Geometry check sheet. Reference: the model listing, model coordinates, mm. Face numbers are marked on the shaded views. A direction names the side the tool comes from. Round coordinates to 2 decimals unless told otherwise and drop trailing zeros. Loops run counter-clockwise (first coordinate to the right, second up) from the corner with the lowest first, then second, coordinate; pieces in that order, holes last. Notation, with made-up numbers: M 2,26.5 L 39,26.5 A30 ccw 39,59.5 Z; hole C -32.5,-36.5 d9. An arc over 180 degrees is marked long. Use one line per item in the form item = value. Start each with the question number.
1. Material ranges on line 1 (Y direction, x = -5, z = 0); line 2 (Y direction, x = -14, z = -3); line 3 (Y direction, x = -15.5, z = 13), recorded low to high.
2. Go/stop test with flat-tipped pins: pin 1 (4 mm diameter, centred on x = -11, y = 40.5, fed in from +Z); pin 2 (6 mm diameter, centred on y = 45, z = -4, fed in from -X); pin 3 (6.5 mm diameter, centred on x = -2.5, y = 44, fed in from -Z). Record where each tip stops, or that it passes through.
3. Cross-section at B-B (x = 15). Record the boundary of the cut face in (y, z).
4. Draft check along Y on the marked faces 1, 2, 3 and 4. Enter one of: pulls with the +Y half, pulls with the -Y half, needs draft (parallel to the pull), parting line crosses it, or undercut.
5. Cross-section at A-A (z = 0.5). Record the boundary of the cut face in (x, y), then the cut area to 3 significant figures.
6. Cross-section at D-D (z = -11.5). Record the boundary of the cut face in (x, y), then the cut area to 3 significant figures.
7. Set-up check for the marked faces 5, 6 and 7: record each of +Z, -Z, +X, -X, +Y, -Y from which the full face is reachable in a straight line by a thin tool's end or side.
8. Cross-section at C-C (y = 13.5). Record the boundary of the cut face in (x, z), then the cut area to 3 significant figures.
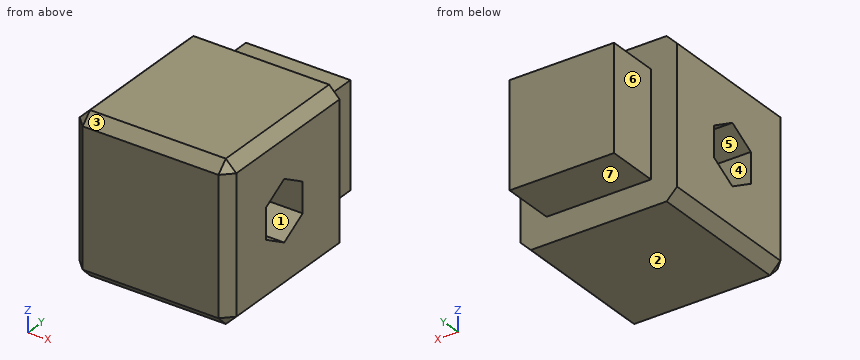
```python
from build123d import *

# Parameters (mm, degrees)
SKETCH1_W           = 38.1
SKETCH1_H           = 38.1
BOSS_EXTRUDE1_DEPTH = 50.8
SKETCH2_W           = 38.1
SKETCH2_H           = 38.1
SKETCH2_W_2         = 25.4
SKETCH2_H_2         = 25.4
CUT_EXTRUDE1_DEPTH  = 12.7
CUT_EXTRUDE2_DEPTH  = 67.295946332
CHAMFER1_SIZE       = 2.54


with BuildPart() as part:
    # Sketch1 → Boss-Extrude1 (new body)
    with BuildSketch(Plane(origin=(0, 0, 0), x_dir=(1, 0, 0), z_dir=(0, 1, 0))):
        Rectangle(SKETCH1_W, SKETCH1_H)
    extrude(amount=BOSS_EXTRUDE1_DEPTH)

    # Sketch2 → Cut-Extrude1 (cut)
    with BuildSketch(Plane(origin=(0, 50.8, 0), x_dir=(1, 0, 0), z_dir=(0, 1, 0))):
        Rectangle(SKETCH2_W, SKETCH2_H)
        Rectangle(SKETCH2_W_2, SKETCH2_H_2, mode=Mode.SUBTRACT)
    extrude(amount=-CUT_EXTRUDE1_DEPTH, mode=Mode.SUBTRACT)

    # Sketch3 → Cut-Extrude2 (cut, through all)
    with BuildSketch(Plane(origin=(19.05, 0, 0), x_dir=(0, 0, -1), z_dir=(1, 0, 0))):
        Polygon((-7.332348419, 19.05), (-3.666174209, 12.7), (3.666174209, 12.7), (7.332348419, 19.05), (3.666174209, 25.4), (-3.666174209, 25.4), align=None)
    extrude(amount=-CUT_EXTRUDE2_DEPTH, mode=Mode.SUBTRACT)

    # Chamfer1
    chamfer1_edges = [part.edges().sort_by_distance(p)[0] for p in [
        (19.05, 19.05, 19.05),
        (-19.05, 19.05, 19.05),
        (-19.05, 19.05, -19.05),
        (19.05, 19.05, -19.05),
        (0, 0, 19.05),
        (-19.05, 0, 0),
        (0, 0, -19.05),
        (19.05, 0, 0),
    ]]
    chamfer(chamfer1_edges, length=CHAMFER1_SIZE)


solid = part.part
```
Reported:
q1.line_1 = 0 to 12.7, 25.4 to 50.8
q1.line_2 = 0 to 12.7, 25.4 to 38.1
q1.line_3 = 0 to 38.1
q2.pin_1 = 12.7
q2.pin_2 = -12.7
q2.pin_3 = -12.7
q3.outline = M 0,-16.51 L 2.54,-19.05 L 38.1,-19.05 L 38.1,19.05 L 2.54,19.05 L 0,16.51 Z; hole M 12.7,-3.67 L 19.05,-7.33 L 25.4,-3.67 L 25.4,3.67 L 19.05,7.33 L 12.7,3.67 Z
q4.face_1 = undercut
q4.face_2 = needs draft
q4.face_3 = pulls with the -Y half
q4.face_4 = undercut
q5.outline = M -19.05,2.54 L -16.51,0 L 16.51,0 L 19.05,2.54 L 19.05,12.7 L -19.05,12.7 Z; M -19.05,25.4 L 19.05,25.4 L 19.05,38.1 L 12.7,38.1 L 12.7,50.8 L -12.7,50.8 L -12.7,38.1 L -19.05,38.1 Z
q5.area = 1,280 mm²
q6.outline = M -19.05,2.54 L -16.51,0 L 16.51,0 L 19.05,2.54 L 19.05,38.1 L 12.7,38.1 L 12.7,50.8 L -12.7,50.8 L -12.7,38.1 L -19.05,38.1 Z
q6.area = 1,770 mm²
q7.face_5 = +X, -X
q7.face_6 = +Z, -Z, -X, +Y
q7.face_7 = -Z, +X, -X, +Y
q8.outline = M -19.05,-16.51 L -16.51,-19.05 L 16.51,-19.05 L 19.05,-16.51 L 19.05,-4.13 L -19.05,-4.13 Z; M -19.05,4.13 L 19.05,4.13 L 19.05,16.51 L 16.51,19.05 L -16.51,19.05 L -19.05,16.51 Z
q8.area = 1,120 mm²
